```python
from build123d import *

# Parameters (mm, degrees)
F1_DEPTH = 12
F2_R     = 1.5
F3_DEPTH = 50
F4_R     = 10
F5_R     = 2


with BuildPart() as f1:
    # F0 (on Top) → F1 (new body)
    with BuildSketch(Plane.XY):
        with BuildLine():
            ThreePointArc((-14.954078, -6.973201), (-3.571254, 16.108884), (16.5, 0))
            Line((16.5, 0), (116.5, 0))
            Line((116.5, 0), (116.5, 15))
            Line((116.5, 15), (27.699278, 15))
            ThreePointArc((27.699278, 15), (-14.162607, 28.136641), (-28.548695, -13.312475))
            Line((-28.548695, -13.312475), (-14.954078, -6.973201))
        make_face()
    extrude(amount=F1_DEPTH)

    # F2 (on Right) → F3 (cut)
    with BuildSketch(Plane.YZ):
        with Locations((0, 6)):
            Circle(F2_R)
    extrude(amount=-F3_DEPTH, mode=Mode.SUBTRACT)

    # F4
    f4_edges = [f1.edges().sort_by_distance(p)[0] for p in [
        (27.699278, 15, 6),
    ]]
    fillet(f4_edges, radius=F4_R)

    # F5
    f5_edges = [f1.edges().sort_by_distance(p)[0] for p in [
        (-16.233753, 26.994727, 12),
        (74.812382, 15, 12),
        (66.5, 0, 12),
        (116.5, 7.5, 12),
        (66.5, 0, 0),
        (116.5, 0, 6),
        (-16.233753, 26.994727, 0),
        (-28.548695, -13.312475, 6),
        (74.812382, 15, 0),
        (116.5, 7.5, 0),
        (116.5, 15, 6),
        (-21.751387, -10.142838, 0),
        (-21.751387, -10.142838, 12),
        (-14.954078, -6.973201, 6),
        (16.5, 0, 6),
    ]]
    fillet(f5_edges, radius=F5_R)


solid = f1.part
```
For this review, take the finished solid that the model builds, in its own axes (mm). A direction names the side the tool comes from. Round coordinates to 2 decimals unless told otherwise and drop trailing zeros. Write each loop counter-clockwise with the first axis right and the second up, starting at its lowest first coordinate (ties: lowest second). Pieces come first, ordered by that corner, then holes. Notation, with made-up numbers: M -26,27 L 6,27 A10 ccw 6,40 Z; hole C 86,-5 d3. An arc over 180 degrees is marked long. One line per item, written item: value. Start each with the question number.
(1) We need section A-A (x = 80.5). Give the boundary of the cut face in (y, z).
(2) Wall thickness on line 1 (Z direction, x = -25.5, y = 0); line 2 (Y direction, x = 95.5, z = 7.75); line 3 (Y direction, x = 0, z = 3.5): over which ranges is each line inside the solid? List them lowest first.
(3) Insertion check: pin 1 (1.8 mm diameter, centred on y = 0, z = 6, fed in from +X); pin 2 (4 mm diameter, centred on y = 22.5, z = 9, fed in from +X); pin 3 (4 mm diameter, centred on y = -3.5, z = 6.5, fed in from -X); pin 4 (20 mm diameter, centred on x = 0, y = 0, fed in from -Z). Each pin has a flat end and moves straight along its axis. Give the tip position at first contact, or say it passes through.
(4) We need section B-B (z = 6). Give the boundary of the cut face in (x, y), and give its area (3 significant figures).
(5) The part is to be moulded in two halves that separate along Y. For faces 4 (the flat face through (31, 10, 0)), 5 (the cylindrical face through (-23.86, -0.325, 4.536)), 6 (the cylindrical face through (-28.29, -12.47, 6.06)), say which applies: released by +Y, released by -Y, zero draft, split by the parting line, or undercut.
(6) Machinability: for faces 1 (the cylindrical face through (-3.95, 16.02, 5.92)), 2 (the flat face through (66, 0, 6)), 3 (the flat face through (74, 15, 6)), which of the approach directions +Z, -Z, +X, -X, +Y, -Y give a long, thin tool a straight path to every point of the face, cutting with its end or side? Answer none if there is none.
Result:
1. outline: M 0,2 A2 ccw 2,0 L 13,0 A2 ccw 15,2 L 15,10 A2 ccw 13,12 L 2,12 A2 ccw 0,10 Z
2. line 1: 0 to 4.5, 7.5 to 12
2. line 2: 0 to 15
2. line 3: 16.5 to 31.5
3. pin 1: x = 116.17
3. pin 2: x = 23.92
3. pin 3: x = -31.46
3. pin 4: through
4. outline: M -31.46,-1.5 A31.5 ccw -29.39,-11.35 A2 ccw -26.67,-12.44 L -16.67,-7.77 A2 ccw -15.62,-5.32 A16.5 cw -16.43,-1.5 Z; M -31.46,1.5 L -16.43,1.5 A16.5 cw 16.4,1.78 A2 ccw 18.39,0 L 114.5,0 A2 ccw 116.5,2 L 116.5,13 A2 ccw 114.5,15 L 33.12,15 A10 cw 25.14,18.98 A31.5 ccw Z
4. area: 2,540 mm²
5. face 4: zero draft
5. face 5: undercut
5. face 6: released by -Y
6. face 1: +Z, -Z
6. face 2: +Z, -Z, +X, -Y
6. face 3: +Z, -Z, +X, +Y
